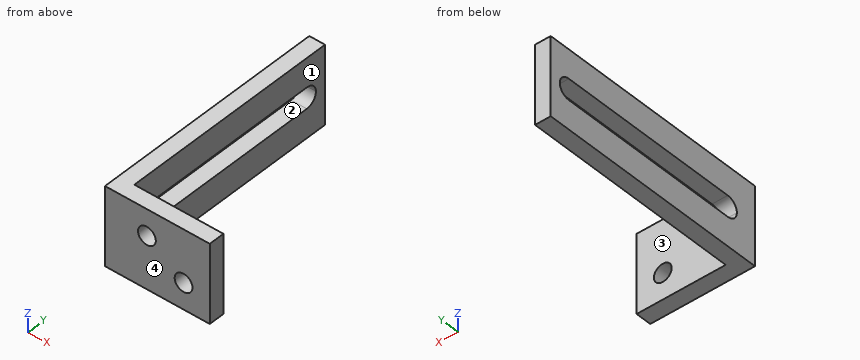
```python
from build123d import *

# Parameters (mm, degrees)
BOSS_EXTRUDE1_DEPTH = 15
CUT_EXTRUDE1_DEPTH  = 6
CUT_EXTRUDE2_REACH  = 50.877
SKETCH3_R           = 1.7


with BuildPart() as part:
    # Sketch1 → Boss-Extrude1 (new body)
    with BuildSketch(Plane.XY):
        Polygon((3, 45), (3, 3), (20, 3), (20, 0), (0, 0), (0, 45), align=None)
    extrude(amount=BOSS_EXTRUDE1_DEPTH)

    # Sketch2 → Cut-Extrude1 (cut)
    with BuildSketch(Plane.ZY):
        with BuildLine():
            ThreePointArc((5.5, 6), (6.085786438, 4.585786438), (7.5, 4))
            Line((7.5, 4), (7.5, 8))
            ThreePointArc((7.5, 8), (6.085786438, 7.414213562), (5.5, 6))
        make_face()
        with BuildLine():
            Line((7.5, 8), (7.5, 4))
            ThreePointArc((7.5, 4), (8.914213562, 4.585786438), (9.5, 6))
            ThreePointArc((9.5, 6), (8.914213562, 7.414213562), (7.5, 8))
        make_face()
        with BuildLine():
            ThreePointArc((5.5, 41), (6.085786438, 39.585786438), (7.5, 39))
            Line((7.5, 39), (7.5, 43))
            ThreePointArc((7.5, 43), (6.085786438, 42.414213562), (5.5, 41))
        make_face()
        with BuildLine():
            Line((7.5, 43), (7.5, 39))
            ThreePointArc((7.5, 39), (8.914213562, 39.585786438), (9.5, 41))
            ThreePointArc((9.5, 41), (8.914213562, 42.414213562), (7.5, 43))
        make_face()
        with BuildLine():
            ThreePointArc((5.5, 6), (6.085786438, 7.414213562), (7.5, 8))
            Line((7.5, 8), (7.5, 39))
            ThreePointArc((7.5, 39), (6.085786438, 39.585786438), (5.5, 41))
            Line((5.5, 41), (5.5, 6))
        make_face()
        with BuildLine():
            Line((7.5, 39), (7.5, 8))
            ThreePointArc((7.5, 8), (8.914213562, 7.414213562), (9.5, 6))
            Line((9.5, 6), (9.5, 41))
            ThreePointArc((9.5, 41), (8.914213562, 39.585786438), (7.5, 39))
        make_face()
    extrude(amount=-CUT_EXTRUDE1_DEPTH, mode=Mode.SUBTRACT)

    # Sketch3 → Cut-Extrude2 (cut, up to next)
    with BuildSketch(Plane(origin=(0, 3, 0), x_dir=(1, 0, 0), z_dir=(0, 1, 0)), mode=Mode.PRIVATE) as cut_extrude2_sk1:
        with Locations(Location((8, -10, 0), (0, 0, 270))):
            Circle(SKETCH3_R)
    cut_extrude2_tool1 = extrude(cut_extrude2_sk1.sketch, amount=-CUT_EXTRUDE2_REACH, mode=Mode.PRIVATE) & part.part
    # Sketch3 → Cut-Extrude2 (cut, up to next)
    with BuildSketch(Plane(origin=(0, 3, 0), x_dir=(1, 0, 0), z_dir=(0, 1, 0)), mode=Mode.PRIVATE) as cut_extrude2_sk2:
        with Locations(Location((15, -5, 0), (0, 0, 270))):
            Circle(SKETCH3_R)
    cut_extrude2_tool2 = extrude(cut_extrude2_sk2.sketch, amount=-CUT_EXTRUDE2_REACH, mode=Mode.PRIVATE) & part.part
    add(cut_extrude2_tool1.solids().sort_by_distance((8, 3, 10))[0], mode=Mode.SUBTRACT)
    add(cut_extrude2_tool2.solids().sort_by_distance((15, 3, 5))[0], mode=Mode.SUBTRACT)


solid = part.part
```
Verification items for the finished model (mm, model axes). Face numbers are marked on the shaded views. Coordinates: 2 decimals unless noted, no trailing zeros. Loops run counter-clockwise (first coordinate to the right, second up) from the corner with the lowest first, then second, coordinate; pieces in that order, holes last. Notation, with made-up numbers: (-34.5, -34.5) - (2.5, -34.5) arc R18 ccw to (2.5, -27.5) - close; hole circle Ø2 at (-2, -37.5). An arc over 180 degrees is marked (long way). Answer as a JSON object with one key per item and string values.
(1) Mould release check, pull along Y, two halves, no side actions. Record for the marked faces 1, 2, 3 and 4: pulls with the +Y half, pulls with the -Y half, needs draft (parallel to the pull), parting line crosses it, or undercut.
Response:
{"face 1": "needs draft", "face 2": "undercut", "face 3": "pulls with the +Y half", "face 4": "pulls with the -Y half"}
(2) Cross-section at C-C, the plane z = 5. Record the boundary of the cut face in (x, y), then the cut area to 3 significant figures.
Response:
{"outline": "(0, 0) - (13.3, 0) - (13.3, 3) - (3, 3) - (3, 45) - (0, 45) - close; (16.7, 0) - (20, 0) - (20, 3) - (16.7, 3) - close", "area": "176 mm²"}
(3) Cross-section at B-B, the plane x = 15. Record the boundary of the cut face in (y, z).
Response:
{"outline": "(0, 0) - (3, 0) - (3, 3.3) - (0, 3.3) - close; (0, 6.7) - (3, 6.7) - (3, 15) - (0, 15) - close"}
(4) Cross-section at A-A, the plane y = 10. Record the boundary of the cut face in (x, z), then the cut area to 3 significant figures.
Response:
{"outline": "(0, 0) - (3, 0) - (3, 5.5) - (0, 5.5) - close; (0, 9.5) - (3, 9.5) - (3, 15) - (0, 15) - close", "area": "33.0 mm²"}
(5) Scan lines: line 1 along Z through (x, y) = (1, 20.5); line 2 along X through (y, z) = (0.8, 10); line 3 along Y through (x, z) = (8.5, 5.5). Record each from-to range of solid material in increasing order.
Response:
{"line 1": "z = 0 to 5.5, 9.5 to 15", "line 2": "x = 0 to 6.3, 9.7 to 20", "line 3": "y = 0 to 3"}
(6) Cross-section at D-D, the plane x = 2.5. Record the boundary of the cut face in (y, z).
Response:
{"outline": "(0, 0) - (45, 0) - (45, 15) - (0, 15) - close; hole (6, 5.5) - (41, 5.5) arc R2 ccw to (41, 9.5) - (6, 9.5) arc R2 ccw to start"}
(7) Go/stop test with a flat-tipped pin: pin 1 Ø5.5 at (x, z) = (15, 5) entering from +Y. Record where the tip stops, or that it passes through.
Response:
{"pin 1": "stops at y = 3"}
